Design review of the part built by this model. Coordinates are the model's own, in mm. Face numbers are marked on the shaded views. A direction names the side the tool comes from. Give positions to 0.01 mm unless a question says otherwise; leave off trailing zeros. Write each loop counter-clockwise with the first axis right and the second up, starting at its lowest first coordinate (ties: lowest second). Pieces come first, ordered by that corner, then holes. Notation, with made-up numbers: (-25, -2) -> (-12, -2) arc R12 ccw to (-12, 8) -> close; hole circle Ø3 at (-11, 69). An arc over 180 degrees is marked (long way). Answer as a JSON object with one key per item and string values.
```python
from build123d import *

# Parameters (mm, degrees)
SKETCH_2_R          = 4.5
EXTRUDE_1_DEPTH     = 10
EXTRUDE_2_DEPTH     = 4
SKETCH_12_R         = 0.8
CUT_EXTRUDE_2_DEPTH = 8
SKETCH_13_R         = 3
EXTRUDE_3_DEPTH     = 2
SKETCH_19_R         = 2.5
EXTRUDE_5_DEPTH     = 5


with BuildPart() as part:
    # 草图2 → 凸台-拉伸1 (new body)
    with BuildSketch(Plane.XY):
        with BuildLine():
            Line((7.102160211, -15.616687508), (44.391240582, 21.672392863))
            ThreePointArc((44.391240582, 21.672392863), (45.562813457, 24.500819988), (44.391240582, 27.329247112))
            Line((44.391240582, 27.329247112), (34.138192255, 37.58229544))
            ThreePointArc((34.138192255, 37.58229544), (31.30976513, 38.753868315), (28.481338005, 37.58229544))
            Line((28.481338005, 37.58229544), (9.215390399, 18.316347834))
            ThreePointArc((9.215390399, 18.316347834), (8.067593218, 16.131525495), (8.362136672, 13.681192624))
            ThreePointArc((8.362136672, 13.681192624), (9.134610316, 6.948541986), (5.886174479, 1.001024456))
            ThreePointArc((5.886174479, 1.001024456), (-7.225109998, -13.84439598), (-17.685225472, -30.663381468))
            ThreePointArc((-17.685225472, -30.663381468), (-11.168239652, -44.207967845), (0.129369861, -34.293788928))
            ThreePointArc((0.129369861, -34.293788928), (1.585802578, -24.197384934), (7.102160211, -15.616687508))
        make_face()
        with Locations((-9.283850525, -34.961173895)):
            Circle(SKETCH_2_R, mode=Mode.SUBTRACT)
        Polygon((39.229361079, 23.581581172), (22.6830624, 7.035282492), (13.844227635, 15.874117257), (30.390526315, 32.420415937), align=None, mode=Mode.SUBTRACT)
    extrude(amount=EXTRUDE_1_DEPTH)

    # 草图4 → 凸台-拉伸2 (add, symmetric)
    with BuildSketch(Plane(origin=(3.298406554, -3.298406554, 0), x_dir=(0, 0, -1), z_dir=(0.7071067811865492, -0.7071067811865458, 0))):
        with BuildLine():
            Line((-9.697397979, 20.014043199), (-9.697397979, 17.014043199))
            Line((-9.697397979, 17.014043199), (-17.697397979, 17.014043199))
            ThreePointArc((-17.697397979, 17.014043199), (-20.525825104, 18.185616074), (-21.697397979, 21.014043199))
            Line((-21.697397979, 21.014043199), (-21.697397979, 45.014043199))
            ThreePointArc((-21.697397979, 45.014043199), (-20.525825104, 47.842470323), (-17.697397979, 49.014043199))
            Line((-17.697397979, 49.014043199), (-9.697397979, 49.014043199))
            Line((-9.697397979, 49.014043199), (-9.697397979, 46.014043199))
            Line((-9.697397979, 46.014043199), (-16.697397979, 46.014043199))
            Line((-16.697397979, 46.014043199), (-16.697397979, 20.014043199))
            Line((-16.697397979, 20.014043199), (-9.697397979, 20.014043199))
        make_face()
    extrude(amount=EXTRUDE_2_DEPTH, both=True)

    # 草图12 → 切除-拉伸2 (cut)
    with BuildSketch(Plane(origin=(0, 0, 0), x_dir=(-1, 0, 0), z_dir=(0, 0, -1))):
        with Locations((-16.354456708, 9.7576436)):
            Circle(SKETCH_12_R)
        with Locations((-36.506999972, 29.910186864)):
            Circle(SKETCH_12_R)
    extrude(amount=-CUT_EXTRUDE_2_DEPTH, mode=Mode.SUBTRACT)

    # 草图13 → 凸台-拉伸3 (add)
    with BuildSketch(Plane.XY.offset(21.697397979)):
        with Locations(Location((30.461236993, 23.864423885, 0), (0, 0, 180))):
            Circle(SKETCH_13_R)
    extrude(amount=EXTRUDE_3_DEPTH)

    # 草图19 → 凸台-拉伸5 (add)
    with BuildSketch(Plane.XY.offset(23.697397979)):
        with Locations((30.461236993, 23.864423885)):
            Circle(SKETCH_19_R)
    extrude(amount=EXTRUDE_5_DEPTH)


solid = part.part
```
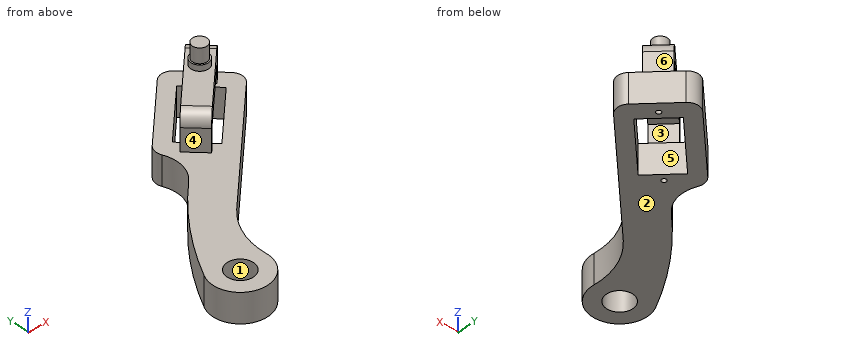
(1) For the marked faces 4, 5 and 6, list the 3-axis set-ups (+Z, -Z, +X, -X, +Y, -Y) from which the entire face can be reached by the end or side of a thin tool; tool diameter is ignored.
Here are the results:
{"face 4": "+Z, -X, -Y", "face 5": "-Z", "face 6": "+Z, +X, +Y"}
(2) We need section C-C, the plane z = 4.5. State the section outline as (x, y) points, then the cut area to 3 significant figures.
Here are the results:
{"outline": "(-17.69, -30.66) arc R9.44 ccw (long way) to (0.13, -34.29) arc R24.01 cw to (7.1, -15.62) -> (44.39, 21.67) arc R4 ccw to (44.39, 27.33) -> (34.14, 37.58) arc R4 ccw to (28.48, 37.58) -> (9.22, 18.32) arc R4.15 ccw to (8.36, 13.68) arc R11.21 cw to (5.89, 1) arc R118.69 ccw to start; hole circle Ø9 at (-9.28, -34.96); hole (13.84, 15.87) -> (22.68, 7.04) -> (39.23, 23.58) -> (30.39, 32.42) -> close; hole circle Ø1.6 at (16.35, 9.76); hole circle Ø1.6 at (36.51, 29.91)", "area": "1,240 mm²"}
(3) For line 1 along Y through (x, z) = (26, 9); line 2 along Z through (x, y) = (11, 2); line 3 along X through (y, z) = (20.5, 3.5), list the stretches that pass through material, from the lowest coordinate up.
Here are the results:
{"line 1": "y = 3.28 to 10.35, 28.03 to 35.1", "line 2": "z = 0 to 10", "line 3": "x = 11.4 to 18.47, 36.15 to 43.22"}
(4) We need section D-D, the plane x = -1. State the section outline as (y, z) points.
Here are the results:
{"outline": "(-39.48, 0) -> (-6.17, 0) -> (-6.17, 10) -> (-39.48, 10) -> close"}
(5) Clearance check with flat-ended pins moving along their axes: pin 1 (4 mm diameter, centred on x = 8.5, z = 5, fed in from +Y); pin 2 (11.5 mm diameter, centred on x = -9.28, y = -34.96, fed in from +Z); pin 3 (4 mm diameter, centred on y = -7.5, z = 13, fed in from -X); pin 4 (2 mm diameter, centred on y = 26, z = 8, fed in from -X). State where each tip first meets the part, or that it passes through.
Here are the results:
{"pin 1": "stops at y = 19.6", "pin 2": "stops at z = 10", "pin 3": "passes through", "pin 4": "stops at x = 15.9"}
(6) The part is to be moulded in two halves that separate along Z. For the marked faces 1, 2 and 3, say which applies: +Z half, -Z half, draft (parallel to the pull), parting line (faces both ways), or undercut.
Here are the results:
{"face 1": "draft", "face 2": "-Z half", "face 3": "undercut"}
(7) We need section A-A, the plane z = 13.25. State the section outline as (x, y) points (3 decimals).
Here are the results:
{"outline": "(12.501, 11.561) -> (18.158, 5.904) -> (20.279, 8.025) -> (14.622, 13.682) -> close; (33.007, 32.067) -> (38.664, 26.41) -> (40.785, 28.531) -> (35.128, 34.188) -> close"}
(8) We need section B-B, the plane y = -38.5. State the section outline as (x, z) points.
Here are the results:
{"outline": "(-18.03, 0) -> (-12.06, 0) -> (-12.06, 10) -> (-18.03, 10) -> close; (-6.5, 0) -> (-0.54, 0) -> (-0.54, 10) -> (-6.5, 10) -> close"}
